Read the model definition and answer for the solid it produces. Units are mm, in the model's axes. A direction names the side the tool comes from. Coordinates: 2 decimals unless noted, no trailing zeros. Order: outer loops, then holes, each group sorted by start corner. A loop starts at its lowest first (then second) coordinate and runs counter-clockwise, first axis right, second up.
from build123d import *

# Parameters (mm, degrees)
SKETCH1_W      = 1219.2
SKETCH1_H      = 609.6
EXTRUDE1_DEPTH = 59.944
SKETCH9_W      = 641.290586706
SKETCH9_H      = 96.25128706
EXTRUDE2_DEPTH = 1304.139971926
SKETCH10_R     = 25.4
EXTRUDE3_DEPTH = 1304.139971926


with BuildPart() as part:
    # Sketch1 → Extrude1 (new body)
    with BuildSketch(Plane(origin=(0, 0, 0), x_dir=(1, 0, 0), z_dir=(0, 1, 0))):
        with Locations((558.660869819, -269.436051937)):
            Rectangle(SKETCH1_W, SKETCH1_H)
    extrude(amount=EXTRUDE1_DEPTH)

    # Sketch9 → Extrude2 (cut, through all)
    with BuildSketch(Plane(origin=(0, 59.944, 0), x_dir=(1, 0, 0), z_dir=(0, 1, 0))):
        with Locations((165.530071427, 7.289591593)):
            Rectangle(SKETCH9_W, SKETCH9_H)
    extrude(amount=-EXTRUDE2_DEPTH, mode=Mode.SUBTRACT)

    # Sketch10 → Extrude3 (cut, through all)
    with BuildSketch(Plane(origin=(0, 59.944, 0), x_dir=(1, 0, 0), z_dir=(0, 1, 0))):
        with Locations(Location((175.855747398, -80.741174358, 0), (0, 0, 270))):
            Circle(SKETCH10_R)
        with Locations(Location((535.065992241, -80.741174358, 0), (0, 0, 90))):
            Circle(SKETCH10_R)
    extrude(amount=-EXTRUDE3_DEPTH, mode=Mode.SUBTRACT)


solid = part.part
Q1. Determine the mould class of faces 1 (the flat face through (550, 30, 574.236)), 2 (the cylindrical face through (151.06, 30.39, 75.23)), 3 (the cylindrical face through (509.882, 30.392, 84.048)), 4 (the flat face through (550, 59.944, 265)) for opening direction Z: +Z half, -Z half, draft (parallel to the pull), parting line (faces both ways), or undercut.
Q2. Which of the six approach directions +Z, -Z, +X, -X, +Y, -Y give full straight-line access (tool end or side, diameter ignored) to faces 5 (the flat face through (822, 30, -35.364)), 6 (the flat face through (214, 30, 40.836))?
Q3. The part is cut by section C-C, the plane y = 50.5. Determine the outline of the cut face in (x, z), then the cut area to 3 significant figures.
Q4. The part is cut by section B-B, the plane z = 68. Determine the outline of the cut face in (x, y), then the cut area to 3 significant figures.
Q5. The part is cut by section A-A, the plane x = 162. Determine the outline of the cut face in (y, z), then the cut area to 3 significant figures.
Q6. Each of these flat-tipped pins is pushed along its axis until it touches: P1, Ø12, axis at x = 664, z = 180.5, coming from the -Y side; P2, Ø2, axis at y = 53, z = 29.5, coming from the -X side. Where does it stop, or does it pass through?
Q7. The part is cut by section D-D, the plane x = 394. Determine the outline of the cut face in (y, z), then the cut area to 3 significant figures.
Q8. Straight lines are drawn through the part: L1, parallel to X at y = 17.5, z = 90.5; L2, parallel to Z at x = 136, y = 42; L3, parallel to Z at x = 523, y = 55.5. For each, find the intervals that lie inside material, in ascending order.
Computed values:
1. face 1: +Z half
1. face 2: undercut
1. face 3: undercut
1. face 4: draft
2. face 5: -Z, +X, -X, +Y, -Y
2. face 6: -Z, -X, +Y, -Y
3. outline: (-50.94, 40.84) - (486.18, 40.84) - (486.18, -35.36) - (1168.26, -35.36) - (1168.26, 574.24) - (-50.94, 574.24) - close; hole circle Ø50.8 at (175.86, 80.74); hole circle Ø50.8 at (535.07, 80.74)
3. area: 698,000 mm2
4. outline: (-50.94, 0) - (153.88, 0) - (153.88, 59.94) - (-50.94, 59.94) - close; (197.83, 0) - (513.09, 0) - (513.09, 59.94) - (197.83, 59.94) - close; (557.04, 0) - (1168.26, 0) - (1168.26, 59.94) - (557.04, 59.94) - close
4. area: 67,800 mm2
5. outline: (0, 40.84) - (59.94, 40.84) - (59.94, 59.45) - (0, 59.45) - close; (0, 102.03) - (59.94, 102.03) - (59.94, 574.24) - (0, 574.24) - close
5. area: 29,400 mm2
6. P1: stops at y = 0
6. P2: stops at x = 486.18
7. outline: (0, 40.84) - (59.94, 40.84) - (59.94, 574.24) - (0, 574.24) - close
7. area: 32,000 mm2
8. L1: x = -50.94 to 152.41, 199.31 to 511.62, 558.52 to 1168.26
8. L2: z = 40.84 to 574.24
8. L3: z = -35.36 to 58.39, 103.09 to 574.24
